The model under review builds one solid part; all positions refer to its coordinate system, in mm. A direction names the side the tool comes from. Round coordinates to 2 decimals unless told otherwise and drop trailing zeros. Write each loop counter-clockwise with the first axis right and the second up, starting at its lowest first coordinate (ties: lowest second). Pieces come first, ordered by that corner, then holes. Notation, with made-up numbers: M 69,-22.75 L 116,-22.75 A24 ccw 116,-12.75 Z; hole C -33.75,74 d8. An arc over 180 degrees is marked long. One line per item, written item: value. Start each with the question number.
1) Wall thickness on probe 1 along Z at (x, y) = (-8, 3.5); probe 2 along Y at (x, z) = (-3, 64): over which ranges is each line inside the solid? List them lowest first.
2) Mouldability with a two-part tool opening along X and no side actions: class faces 1 (the face through (0, 18, 148)), 2 (the face through (-20, 0, 320)), 3 (the face through (0, 0, 302)) as +X half, -X half, draft (parallel to the pull), parting line (faces both ways), or undercut.
3) Take a section at C-C, the plane z = 227.5. Write out the cut boundary in (x, y), and give its area (3 significant figures).
4) Take a section at A-A, the plane y = 11.5. Write out the cut boundary in (x, z), and give its area (3 significant figures).
5) Tool access review of faces 4 (the face through (-18, 0, 148)), 5 (the face through (18, 0, 320)), 6 (the face through (0, 0, 0)), 7 (the face through (0, -18, 148)), 8 (the face through (18, 0, 148)): name each direction out of +Z, -Z, +X, -X, +Y, -Y from which nothing blocks a thin tool from reaching the whole face with its end or side.
6) Take a section at B-B, the plane x = 9.5. Write out the cut boundary in (y, z).
7) For P1, Ø3, axis at x = 6, z = 281, coming from the -Y side; P2, Ø12, axis at x = -15, z = 138, coming from the +Y side; P3, Ø3, axis at y = -16, z = 72.5, coming from the -X side, all flat-tipped, find the tip position at first contact; note any pin that passes through.
from build123d import *

# Parameters (mm, degrees)
SKETCH1_W                = 36
SKETCH1_H                = 36
BOSS_EXTRUDE1_DEPTH      = 300
BOSS_EXTRUDE2_DEPTH      = 20
BOSS_EXTRUDE2_DEPTH_BACK = 20
SKETCH2_W                = 40
SKETCH2_H                = 40
SKETCH2_W_2              = 36
SKETCH2_H_2              = 36


with BuildPart() as part:
    # Sketch1 → Boss-Extrude1 (new body)
    with BuildSketch(Plane.XY):
        Rectangle(SKETCH1_W, SKETCH1_H)
    extrude(amount=BOSS_EXTRUDE1_DEPTH)

    # Sketch2 → Boss-Extrude2 (add, two sides: drawn at the far end of the back side and taken through both)
    with BuildSketch(Plane(origin=(0, 0, 0), x_dir=(1, 0, 0), z_dir=(0, 1, 0)).offset(-BOSS_EXTRUDE2_DEPTH_BACK)):
        with Locations((0, -320)):
            Rectangle(SKETCH2_W, SKETCH2_H)
        with Locations((0, -320)):
            Rectangle(SKETCH2_W_2, SKETCH2_H_2, mode=Mode.SUBTRACT)
    extrude(amount=BOSS_EXTRUDE2_DEPTH + BOSS_EXTRUDE2_DEPTH_BACK)


solid = part.part
Checked values:
1. probe 1: z = 0 to 302, 338 to 340
1. probe 2: y = -18 to 18
2. face 1: draft
2. face 2: -X half
2. face 3: undercut
3. outline: M -18,-18 L 18,-18 L 18,18 L -18,18 Z
3. area: 1,300 mm2
4. outline: M -20,300 L -18,300 L -18,0 L 18,0 L 18,300 L 20,300 L 20,340 L -20,340 Z; hole M -18,302 L 18,302 L 18,338 L -18,338 Z
4. area: 11,100 mm2
5. face 4: -Z, -X, +Y, -Y
5. face 5: +Y, -Y
5. face 6: -Z, +X, -X, +Y, -Y
5. face 7: -Z, +X, -X, -Y
5. face 8: -Z, +X, +Y, -Y
6. outline: M -20,300 L -18,300 L -18,0 L 18,0 L 18,300 L 20,300 L 20,302 L -20,302 Z; M -20,338 L 20,338 L 20,340 L -20,340 Z
7. P1: stops at y = -18
7. P2: stops at y = 18
7. P3: stops at x = -18
